from build123d import *

# Parameters (mm, degrees)
BOSS_EXTRUDE1_DEPTH = 10
CUT_EXTRUDE1_DEPTH  = 68.119296778


with BuildPart() as part:
    # Sketch1 → Boss-Extrude1 (new body)
    with BuildSketch(Plane(origin=(0, 0, 0), x_dir=(1, 0, 0), z_dir=(0, 1, 0))):
        Polygon((0, 0), (-14, 0), (-14, -10), (-24, -10), (-24, 0), (-34, 0), (-34, 10), (0, 57), (0, 44.2), (10, 44.2), (10, 34.2), (0, 34.2), (0, 22.2), (10, 22.2), (10, 12.2), (0, 12.2), align=None)
    extrude(amount=BOSS_EXTRUDE1_DEPTH)

    # Sketch3 → Cut-Extrude1 (cut, through all)
    with BuildSketch(Plane(origin=(0, 10, 0), x_dir=(1, 0, 0), z_dir=(0, 1, 0))):
        with BuildLine():
            Line((-11, 29.75), (-8, 29.75))
            Line((-8, 29.75), (-8, 30.55))
            ThreePointArc((-8, 30.55), (-7.853553391, 30.903553391), (-7.5, 31.05))
            Line((-7.5, 31.05), (-5, 31.05))
            ThreePointArc((-5, 31.05), (-4.646446609, 30.903553391), (-4.5, 30.55))
            Line((-4.5, 30.55), (-4.5, 29.75))
            Line((-4.5, 29.75), (0, 29.75))
            Line((0, 29.75), (0, 26.65))
            Line((0, 26.65), (-4.5, 26.65))
            Line((-4.5, 26.65), (-4.5, 25.85))
            ThreePointArc((-4.5, 25.85), (-4.646446609, 25.496446609), (-5, 25.35))
            Line((-5, 25.35), (-7.5, 25.35))
            ThreePointArc((-7.5, 25.35), (-7.853553391, 25.496446609), (-8, 25.85))
            Line((-8, 25.85), (-8, 26.65))
            Line((-8, 26.65), (-11, 26.65))
            Line((-11, 26.65), (-11, 29.75))
        make_face()
    extrude(amount=-CUT_EXTRUDE1_DEPTH, mode=Mode.SUBTRACT)


solid = part.part
The model under review builds one solid part; all positions refer to its coordinate system, in mm. A direction names the side the tool comes from. Round coordinates to 2 decimals unless told otherwise and drop trailing zeros. Order: outer loops, then holes, each group sorted by start corner. A loop starts at its lowest first (then second) coordinate and runs counter-clockwise, first axis right, second up. Notation, with made-up numbers: (66.5, -29.75) -> (84.5, -29.75) arc R22 ccw to (84.5, -18.75) -> close; hole circle Ø1 at (-27.5, 35). An arc over 180 degrees is marked (long way). Write item = value, one per line. Start each with the question number.
Item 1: Mouldability with a two-part tool opening along X and no side actions: class faces 1 (the face through (-34, 5, -5)), 2 (the face through (-6, 5, -25.35)), 3 (the face through (-12, 10, -17)) as released by +X, released by -X, zero draft, split by the parting line, or undercut.
Item 2: Clearance check with flat-ended pins moving along their axes: pin 1 Ø1.5 at (x, y) = (-9.5, 6.5) entering from +Z; pin 2 Ø3 at (y, z) = (5, 3) entering from -X; pin 3 Ø0.6 at (y, z) = (3, -30) entering from +X. State where each tip first meets the part, or that it passes through.
Item 3: For line 1 along X through (y, z) = (4.5, 5); line 2 along Z through (x, y) = (-5, 8.5); line 3 along X through (y, z) = (9.5, -3), list the stretches that pass through material, from the lowest coordinate up.
Item 4: For faces 4 (the face through (5, 5, -12.2)), 5 (the face through (-29, 5, 0)), 6 (the face through (5, 5, -34.2)), list the 3-axis set-ups (+Z, -Z, +X, -X, +Y, -Y) from which the entire face can be reached by the end or side of a thin tool; tool diameter is ignored.
Item 5: Consider section D-D on z = 1.5. Write out the cut boundary in (x, y).
Item 6: Consider section A-A on x = 4. Write out the cut boundary in (y, z), plus the area to 3 significant figures.
Item 7: Consider section C-C on x = -9. Write out the cut boundary in (y, z), plus the area to 3 significant figures.
Conclusion:
q1.face_1 = released by -X
q1.face_2 = undercut
q1.face_3 = zero draft
q2.pin_1 = 0
q2.pin_2 = -24
q2.pin_3 = 0
q3.line_1 = -24 to -14
q3.line_2 = -50.09 to -31.05, -25.35 to 0
q3.line_3 = -34 to 0
q4.face_4 = +Z, +X, +Y, -Y
q4.face_5 = +Z, -X, +Y, -Y
q4.face_6 = +X, +Y, -Y
q5.outline = (-24, 0) -> (-14, 0) -> (-14, 10) -> (-24, 10) -> close
q6.outline = (0, -44.2) -> (10, -44.2) -> (10, -34.2) -> (0, -34.2) -> close; (0, -22.2) -> (10, -22.2) -> (10, -12.2) -> (0, -12.2) -> close
q6.area = 200 mm2
q7.outline = (0, -44.56) -> (10, -44.56) -> (10, -29.75) -> (0, -29.75) -> close; (0, -26.65) -> (10, -26.65) -> (10, 0) -> (0, 0) -> close
q7.area = 415 mm2
